```python
from build123d import *
from build123d.topology import SkipClean

# Parameters (mm, degrees)
BOSS_EXTRUDE1_DEPTH             = 25
BOSS_EXTRUDE2_REACH             = 65.362
BOSS_EXTRUDE2_DIRECTION_2_DEPTH = 30
SKETCH9_R                       = 2.05
CUT_EXTRUDE3_DEPTH              = 35
BOSS_EXTRUDE5_REACH             = 63.601
SKETCH13_R                      = 1.55
CUT_EXTRUDE4_DEPTH              = 88.693844753
SKETCH16_W                      = 63
SKETCH16_H                      = 45
CUT_EXTRUDE5_DEPTH              = 65.196143
BOSS_EXTRUDE6_DEPTH             = 17.5
SKETCH18_R                      = 2.05
CUT_EXTRUDE6_DEPTH              = 17.5


with BuildPart() as part:
    # Sketch1 → Boss-Extrude1 (new, symmetric)
    with BuildSketch(Plane.XY):
        with BuildLine():
            Line((-17.5, 22.5), (-17.5, 0))
            Line((-17.5, 0), (17.5, 0))
            Line((17.5, 0), (17.5, 22.5))
            Line((17.5, 22.5), (12.5, 22.5))
            ThreePointArc((12.5, 22.5), (0, 10), (-12.5, 22.5))
            Line((-12.5, 22.5), (-17.5, 22.5))
        make_face()
    boss_extrude1 = extrude(amount=BOSS_EXTRUDE1_DEPTH, both=True)

    # Boss-Extrude2: up to this face of the body (flat: up to its plane)
    boss_extrude2_end = Plane(part.part.faces().sort_by_distance((17.5, 11.25, 0))[0])
    # Sketch5 → Boss-Extrude2 (add, up to the picked face)
    with BuildSketch(Plane(origin=(26.115381057, 0, 15.077722283), x_dir=(0.500000000000001, 0, -0.8660254037844382), z_dir=(0.8660254037844382, 0, 0.500000000000001)), mode=Mode.PRIVATE) as boss_extrude2_sk1:
        with BuildLine():
            Line((-8.7, 22.5), (-3.75, 22.5))
            ThreePointArc((-3.75, 22.5), (8.75, 10), (21.25, 22.5))
            Line((21.25, 22.5), (26.2, 22.5))
            ThreePointArc((26.2, 22.5), (8.75, 5.05), (-8.7, 22.5))
        make_face()
    boss_extrude2_tool1 = split(extrude(boss_extrude2_sk1.sketch, amount=-BOSS_EXTRUDE2_REACH, mode=Mode.PRIVATE), bisect_by=boss_extrude2_end, keep=Keep.BOTH, mode=Mode.PRIVATE)
    boss_extrude2 = boss_extrude2_tool1.solids().sort_by(Axis((23.002881, 22.109806, 20.46873), (-0.8660254037844382, 0, -0.500000000000001)))[0]
    add(boss_extrude2)

    # Sketch5 → Boss-Extrude2 direction 2 (add)
    with BuildSketch(Plane(origin=(26.115381057, 0, 15.077722283), x_dir=(0.500000000000001, 0, -0.8660254037844382), z_dir=(0.8660254037844382, 0, 0.500000000000001))):
        with BuildLine():
            Line((-8.7, 22.5), (-3.75, 22.5))
            ThreePointArc((-3.75, 22.5), (8.75, 10), (21.25, 22.5))
            Line((21.25, 22.5), (26.2, 22.5))
            ThreePointArc((26.2, 22.5), (8.75, 5.05), (-8.7, 22.5))
        make_face()
    boss_extrude2_direction_2 = extrude(amount=BOSS_EXTRUDE2_DIRECTION_2_DEPTH)

    # Sketch9 → Cut-Extrude3 (cut)
    with BuildSketch(Plane.ZY.offset(17.5)):
        with Locations((-18, 5)):
            Circle(SKETCH9_R)
    cut_extrude3 = extrude(amount=-CUT_EXTRUDE3_DEPTH, mode=Mode.SUBTRACT)

    # Boss-Extrude5: up to this face of the body (flat: up to its plane)
    boss_extrude5_end = Plane(part.part.faces().sort_by_distance((17.5, 17.19483523, 0))[0])
    # Sketch12 → Boss-Extrude5 (add, up to the picked face)
    with BuildSketch(Plane(origin=(21.973076211, 0, 12.686161466), x_dir=(0.4999999999999999, 0, -0.8660254037844388), z_dir=(0.8660254037844388, 0, 0.4999999999999999)), mode=Mode.PRIVATE) as boss_extrude5_sk1:
        with BuildLine():
            Line((-3.75, 22.5), (21.25, 22.5))
            ThreePointArc((21.25, 22.5), (8.75, 10), (-3.75, 22.5))
        make_face()
    boss_extrude5_tool1 = split(extrude(boss_extrude5_sk1.sketch, amount=-BOSS_EXTRUDE5_REACH, mode=Mode.PRIVATE), bisect_by=boss_extrude5_end, keep=Keep.BOTH, mode=Mode.PRIVATE)
    boss_extrude5 = boss_extrude5_tool1.solids().sort_by(Axis((26.348076, 17.194835, 5.108439), (-0.8660254037844388, 0, -0.4999999999999999)))[0]
    add(boss_extrude5)

    # Mirror1: Boss-Extrude1, Boss-Extrude2, Boss-Extrude2 direction 2, Cut-Extrude3, Boss-Extrude5 across plane
    with SkipClean():  # the faces are left unmerged after this step: merging them gives an invalid solid
        add(boss_extrude1.mirror(Plane(origin=(17.5, 22.5, 25), x_dir=(0, 0, 1), z_dir=(0, -1, 0))))
        add(boss_extrude2.mirror(Plane(origin=(17.5, 22.5, 25), x_dir=(0, 0, 1), z_dir=(0, -1, 0))))
        add(boss_extrude2_direction_2.mirror(Plane(origin=(17.5, 22.5, 25), x_dir=(0, 0, 1), z_dir=(0, -1, 0))))
        add(cut_extrude3.mirror(Plane(origin=(17.5, 22.5, 25), x_dir=(0, 0, 1), z_dir=(0, -1, 0))), mode=Mode.SUBTRACT)
        add(boss_extrude5.mirror(Plane(origin=(17.5, 22.5, 25), x_dir=(0, 0, 1), z_dir=(0, -1, 0))))

    # Sketch13 → Cut-Extrude4 (cut, through all)
    with SkipClean():  # the faces are left unmerged after this step: merging them gives an invalid solid
        with BuildSketch(Plane(origin=(0, 0, 0), x_dir=(1, 0, 0), z_dir=(0, 1, 0))):
            with Locations(Location((43.480762114, -15, 0), (0, 0, 90))):
                Circle(SKETCH13_R)
        extrude(amount=CUT_EXTRUDE4_DEPTH, mode=Mode.SUBTRACT)

    # Sketch16 → Cut-Extrude5 (cut)
    with BuildSketch(Plane(origin=(0, 0, 0), x_dir=(0, 0, -1), z_dir=(1, 0, 0))):
        with Locations((-6.5, 22.5)):
            Rectangle(SKETCH16_W, SKETCH16_H)
    extrude(amount=CUT_EXTRUDE5_DEPTH, mode=Mode.SUBTRACT)

    # Sketch17 → Boss-Extrude6 (add)
    with BuildSketch(Plane.ZY.offset(17.5)):
        with BuildLine():
            Line((13, 0), (23, 0))
            ThreePointArc((23, 0), (18, -5), (13, 0))
        make_face()
    boss_extrude6 = extrude(amount=-BOSS_EXTRUDE6_DEPTH)

    # Sketch18 → Cut-Extrude6 (cut)
    with BuildSketch(Plane.ZY.offset(17.5)):
        with Locations(Location((18, 0, 0), (0, 0, 270))):
            Circle(SKETCH18_R)
    cut_extrude6 = extrude(amount=-CUT_EXTRUDE6_DEPTH, mode=Mode.SUBTRACT)

    # Mirror2: Boss-Extrude6, Cut-Extrude6 across plane
    add(boss_extrude6.mirror(Plane.ZX.offset(22.5)))
    add(cut_extrude6.mirror(Plane.ZX.offset(22.5)), mode=Mode.SUBTRACT)


solid = part.part
```
Part model, mm, in its own coordinate system. A direction names the side the tool comes from. Coordinates: 2 decimals unless noted, no trailing zeros. Order: outer loops, then holes, each group sorted by start corner. A loop starts at its lowest first (then second) coordinate and runs counter-clockwise, first axis right, second up. Notation, with made-up numbers: (-23.75, 77.5) -> (18.25, 77.5) arc R27 ccw to (18.25, 95.5) -> close; hole circle Ø5 at (-29.5, 28). An arc over 180 degrees is marked (long way). Put each result on its own line as item: value. Start each with the question number.
(1) Pin check, flat tips, straight feed: pin 1 Ø4 at (x, z) = (-6.5, -6.5) entering from +Y; pin 2 Ø6 at (x, z) = (-12.5, -8.5) entering from -Y; pin 3 Ø3.5 at (y, z) = (0, 18) entering from +X. Stop position of each tip, or through.
(2) Band-saw the part on C-C (y = 5). Give the cut face in (x, z), then the cut area to 3 significant figures.
(3) Band-saw the part on D-D (z = -8). Give the cut face in (x, y), then the cut area to 3 significant figures.
(4) Probe line 1 along Z through (x, y) = (-6.25, 40); line 2 along Y through (x, z) = (-9, -18); line 3 along Y through (x, z) = (-7.25, 17.5). List the from-to ranges inside material, lowest first. Write a range as [from, to].
(5) Band-saw the part on A-A (x = -3.5). Give the cut face in (y, z).
(6) Mould opens along Z. For faces 4 (the face through (-8.872, 37.967, -18.267)), 5 (the face through (-9, 45, -6)), 6 (the face through (-9, 50, 18)), 7 (the face through (-8.87, 42.95, 18.09)) say: pulls with the +Z half, pulls with the -Z half, needs draft (parallel to the pull), parting line crosses it, or undercut.
(7) Band-saw the part on B-B (z = 18). Give the cut face in (x, y).
(8) Which spindle directions (+Z, -Z, +X, -X, +Y, -Y) get a long thin tool onto all of the face, cutting with end or side? Do faces 1 (the face through (-9, 0, 24)), 2 (the face through (-9, 0, -6)), 3 (the face through (-9, 45, 24)). Say none if no direction does.
Determined:
1. pin 1: stops at y = 45
1. pin 2: stops at y = 0
1. pin 3: passes through
2. outline: (-17.5, -25) -> (0, -25) -> (0, -20.05) -> (-17.5, -20.05) -> close; (-17.5, -15.95) -> (0, -15.95) -> (0, 25) -> (-17.5, 25) -> close
2. area: 803 mm²
3. outline: (-17.5, 0) -> (0, 0) -> (0, 10) arc R12.5 cw to (0, 35) -> (0, 45) -> (-17.5, 45) -> close
3. area: 542 mm²
4. line 1: z = [-25, -20.05], [-15.95, 25]
4. line 2: y = [0, 2.95], [7.05, 13.83], [31.17, 37.95], [42.05, 45]
4. line 3: y = [-4.97, -1.99], [1.99, 12.32], [32.68, 43.01], [46.99, 49.97]
5. outline: (0, -25) -> (10.5, -25) -> (10.5, 25) -> (0, 25) -> (0, 23) arc R5 ccw to (0, 13) -> close; (34.5, -25) -> (45, -25) -> (45, 13) arc R5 ccw to (45, 23) -> (45, 25) -> (34.5, 25) -> close; hole circle Ø4.1 at (0, 18); hole circle Ø4.1 at (5, -18); hole circle Ø4.1 at (40, -18); hole circle Ø4.1 at (45, 18)
6. face 4: undercut
6. face 5: needs draft
6. face 6: parting line crosses it
6. face 7: undercut
7. outline: (-17.5, -5) -> (0, -5) -> (0, -2.05) -> (-17.5, -2.05) -> close; (-17.5, 2.05) -> (0, 2.05) -> (0, 10) arc R12.5 cw to (0, 35) -> (0, 42.95) -> (-17.5, 42.95) -> close; (-17.5, 47.05) -> (0, 47.05) -> (0, 50) -> (-17.5, 50) -> close
8. face 1: +Z, +X, -X, -Y
8. face 2: -Z, +X, -X, -Y
8. face 3: +Z, +X, -X, +Y
